CAD build for the part. Positions are in the model's coordinates, mm. Give positions to 0.01 mm unless a question says otherwise; leave off trailing zeros. Write each loop counter-clockwise with the first axis right and the second up, starting at its lowest first coordinate (ties: lowest second). Pieces come first, ordered by that corner, then holes. Notation, with made-up numbers: (11.25, -10.75) - (24.25, -10.75) arc R19 ccw to (24.25, 11.25) - close; hole circle Ø9 at (59.25, 47). An arc over 180 degrees is marked (long way). Put each result on its own line as item: value. Start each with the question number.
1. Wall check: line 1 (X direction, y = -35, z = 43); line 2 (Y direction, x = 28, z = 38); line 3 (Y direction, x = 35.5, z = 36.25). Give the ranges that are in metal, low to high.
2. Cut at D-D on z = 42. List the corners of the cut face in (x, y).
3. Cut at A-A on z = 34.5. List the corners of the cut face in (x, y), and give its area (3 significant figures).
4. Cut at B-B on y = -39. List the corners of the cut face in (x, z) (3 decimals).
from build123d import *

# Parameters (mm, degrees)
F0_W     = 63.5
F0_H     = 63.5
F1_DEPTH = 44.45
F5_W     = 63.5
F5_H     = 19.05
F6_DEPTH = 63.501
F7_R     = 5.08


with BuildPart() as f1:
    # F0 (on Top) → F1 (new body)
    with BuildSketch(Plane.XY):
        with Locations((31.75, -31.75)):
            Rectangle(F0_W, F0_H)
    extrude(amount=F1_DEPTH)

    # F3 (on offset) → F4 (revolve, cut)
    with BuildSketch(Plane.XY.offset(60.325)):
        with BuildLine():
            Line((60.325, -31.75), (3.175, -31.75))
            ThreePointArc((3.175, -31.75), (31.75, -60.325), (60.325, -31.75))
        make_face()
    revolve(axis=Axis((31.75, -31.75, 60.325), (1, 0, 0)), mode=Mode.SUBTRACT)

    # F5 (on face) → F6 (cut, through all)
    with BuildSketch(Plane.XZ.offset(63.5)):
        with Locations((31.75, 9.525)):
            Rectangle(F5_W, F5_H)
    extrude(amount=-F6_DEPTH, mode=Mode.SUBTRACT)

    # F7
    f7_edges = [f1.edges().sort_by_distance(p)[0] for p in [
        (63.5, -63.5, 31.75),
        (63.5, 0, 31.75),
        (0, 0, 31.75),
        (0, -63.5, 31.75),
    ]]
    fillet(f7_edges, radius=F7_R)


solid = f1.part
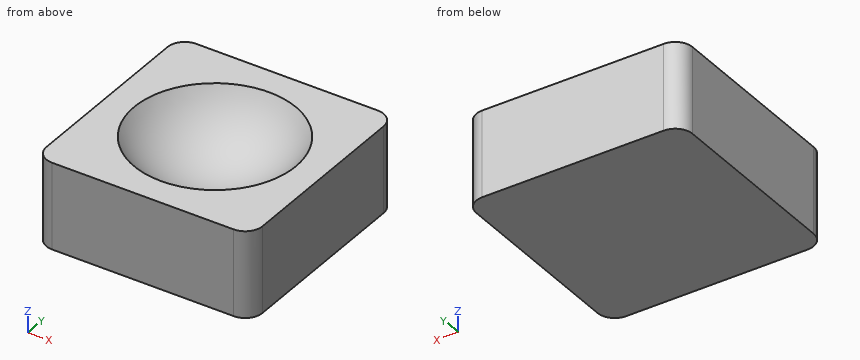
Report:
1. line 1: x = 0 to 9.26, 54.24 to 63.5
1. line 2: y = -63.5 to -49.19, -14.31 to 0
1. line 3: y = -63.5 to -46.68, -16.82 to 0
2. outline: (0, -58.42) arc R5.08 ccw to (5.08, -63.5) - (58.42, -63.5) arc R5.08 ccw to (63.5, -58.42) - (63.5, -5.08) arc R5.08 ccw to (58.42, 0) - (5.08, 0) arc R5.08 ccw to (0, -5.08) - close; hole circle Ø43.85 at (31.75, -31.75)
3. outline: (0, -58.42) arc R5.08 ccw to (5.08, -63.5) - (58.42, -63.5) arc R5.08 ccw to (63.5, -58.42) - (63.5, -5.08) arc R5.08 ccw to (58.42, 0) - (5.08, 0) arc R5.08 ccw to (0, -5.08) - close; hole circle Ø24.46 at (31.75, -31.75)
3. area: 3,540 mm²
4. outline: (0, 19.05) - (63.5, 19.05) - (63.5, 44.45) - (54.376, 44.45) arc R27.64 cw to (9.124, 44.45) - (0, 44.45) - close
